Could you check a few things on this drawing? It's one solid part, dimensions in mm from its lowest x, y, z. Round coordinates to 2 decimals unless told otherwise and drop trailing zeros. Loops run counter-clockwise (first coordinate to the right, second up) from the corner with the lowest first, then second, coordinate; pieces in that order, holes last. Notation, with made-up numbers: M 18,60.5 L 76,60.5 A34 ccw 76,91.5 Z; hole C -36,25.5 d8. An arc over 180 degrees is marked long. Return JSON: item names as keys, results as strings.
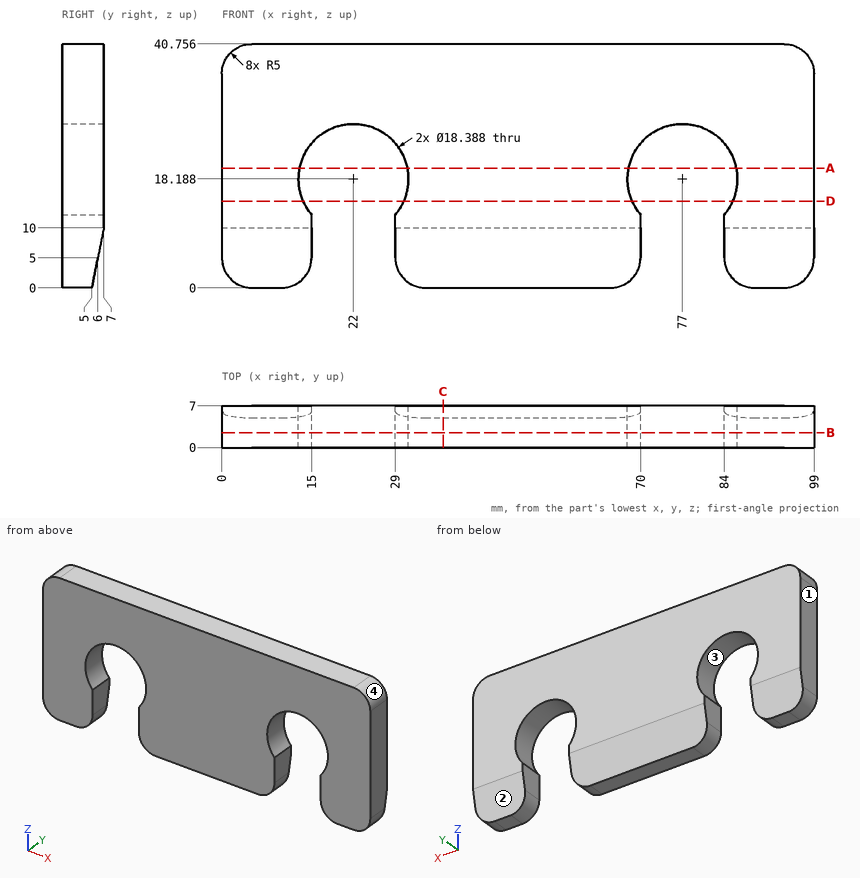
Q1. Suppose I cut it at B-B, the plane y = 2.5. Please give me the cut outline in (x, z) (1 decimal), plus the area to 3 significant figures.
Results:
{"outline": "M 0,5 A5 ccw 5,0 L 10,0 A5 ccw 15,5 L 15,12.2 A9.2 cw long 29,12.2 L 29,5 A5 ccw 34,0 L 65,0 A5 ccw 70,5 L 70,12.2 A9.2 cw long 84,12.2 L 84,5 A5 ccw 89,0 L 94,0 A5 ccw 99,5 L 99,35.8 A5 ccw 94,40.8 L 5,40.8 A5 ccw 0,35.8 Z", "area": "3,180 mm2"}
Q2. If I drill on line 1 along X through (y, z) = (4.25, 12); line 2 along X through (y, z) = (5, 3); line 3 along Z through (x, y) = (22, 4.25) (1 decimal), over which ranges is the centre line in solid material (lowest first)?
Results:
{"line 1": "x = 0 to 15, 29 to 70, 84 to 99", "line 2": "x = 0.42 to 14.58, 29.42 to 69.58, 84.42 to 98.58", "line 3": "z = 27.4 to 40.8"}
Q3. I'm going to push a flat-ended pin straight in: pin 1 Ø14.5 at (x, z) = (22, 18.19) entering from +Y. Where does the tip first touch, or does it pass through?
Results:
{"pin 1": "passes through"}
Q4. Suppose I cut it at D-D, the plane z = 14.5. Please give me the cut outline in (x, y).
Results:
{"outline": "M 0,0 L 13.58,0 L 13.58,7 L 0,7 Z; M 30.42,0 L 68.58,0 L 68.58,7 L 30.42,7 Z; M 85.42,0 L 99,0 L 99,7 L 85.42,7 Z"}
Q5. Thinking about a two-plate mould opening in X: for the marked faces 1, 2, 3 and 4, which applies, pulls with the +X half, pulls with the -X half, needs draft (parallel to the pull), parting line crosses it, or undercut?
Results:
{"face 1": "pulls with the -X half", "face 2": "needs draft", "face 3": "undercut", "face 4": "pulls with the +X half"}
Q6. Suppose I cut it at A-A, the plane z = 20. Please give me the cut outline in (x, y).
Results:
{"outline": "M 0,0 L 12.99,0 L 12.99,7 L 0,7 Z; M 31.01,0 L 67.99,0 L 67.99,7 L 31.01,7 Z; M 86.01,0 L 99,0 L 99,7 L 86.01,7 Z"}
Q7. Suppose I cut it at C-C, the plane x = 37. Please give me the cut outline in (y, z) (1 decimal).
Results:
{"outline": "M 0,0 L 5,0 L 7,10 L 7,40.8 L 0,40.8 Z"}
